```python
from build123d import *

# Parameters (mm, degrees)
F1_DEPTH      = 13
F3_W          = 5.624003956
F3_H          = 13
F4_DEPTH      = 0.5
F6_DEPTH      = 9
F8_W          = 1.375
F8_H          = 2.5
F9_DEPTH      = 0.5
F10_R         = 2
F11_R         = 1
F12_T1_DEPTH  = 14.5
F13_T1_DEPTH  = 0.5
F13_T6_DEPTH  = 0.5
F13_S7_R      = 1.95289555
F13_T8_DEPTH  = 2
F13_T12_DEPTH = 0.5
F13_S13_R     = 1.95289555
F13_T14_DEPTH = 2


# Not quite as in the source:
# - a fillet or chamfer that OpenCascade refuses, or shapes differently, is made with other operations: its cross-section is extruded or revolved along the edge and cut away or added


with BuildPart() as f1:
    # F0 (on Front) → F1 (new body)
    with BuildSketch(Plane.XZ):
        with BuildLine():
            Line((-0.1891016816, 7.3390506263), (-0.5721239031, 7.6604444312))
            Line((-0.5721239031, 7.6604444312), (-4.3080067621, 3.2081926126))
            ThreePointArc((-4.3080067621, 3.2081926126), (-4.5819264222, 1.1275662273), (-2.812001978, 0))
            Line((-2.812001978, 0), (0, 0))
            Line((0, 0), (0, 0.5))
            Line((0, 0.5), (-2.812001978, 0.5))
            ThreePointArc((-2.812001978, 0.5), (-4.1287725287, 1.3388753582), (-3.9249845405, 2.8867988077))
            Line((-3.9249845405, 2.8867988077), (-0.1891016816, 7.3390506263))
        make_face()
        with BuildLine():
            Line((0, 0.5), (0, 0))
            Line((0, 0), (2.812001978, 0))
            ThreePointArc((2.812001978, 0), (4.5819264222, 1.1275662273), (4.3080067621, 3.2081926126))
            Line((4.3080067621, 3.2081926126), (0.5721239031, 7.6604444312))
            Line((0.5721239031, 7.6604444312), (0.1891016816, 7.3390506263))
            Line((0.1891016816, 7.3390506263), (3.9249845405, 2.8867988077))
            ThreePointArc((3.9249845405, 2.8867988077), (4.1287725287, 1.3388753582), (2.812001978, 0.5))
            Line((2.812001978, 0.5), (0, 0.5))
        make_face()
    extrude(amount=-F1_DEPTH)

    # F3 (on offset) → F4 (join, through all)
    with BuildSketch(Plane(origin=(0, 0, 0), x_dir=(1, 0, 0), z_dir=(0, 0, -1))):
        with Locations((0, -6.5)):
            Rectangle(F3_W, F3_H)
        with BuildLine():
            Line((-2.812001978, 0), (2.812001978, 0))
            Line((2.812001978, 0), (4.4072171914, 0.6821090398))
            ThreePointArc((4.4072171914, 0.6821090398), (4.4747132661, 0.7384715991), (4.5, 0.8226917824))
            Line((4.5, 0.8226917824), (4.5, 15))
            Line((4.5, 15), (-4.5, 15))
            Line((-4.5, 15), (-4.5, 0.8226917824))
            ThreePointArc((-4.5, 0.8226917824), (-4.4747132661, 0.7384715991), (-4.4072171914, 0.6821090398))
            Line((-4.4072171914, 0.6821090398), (-2.812001978, 0))
        make_face()
    extrude(amount=-F4_DEPTH)

    # F5 (on face) → F6 (join, through all)
    with BuildSketch(Plane.YZ.offset(4.5)):
        Polygon((-22.4330127019, -11.874355653), (-22, -12.124355653), (-15, 0), (-15, 0.5), (-15.2886751346, 0.5), align=None)
    extrude(amount=-F6_DEPTH)

    # F8 (on offset) → F9 (join, through all)
    with BuildSketch(Plane(origin=(0, -11.6830127019, 6.7451905284), x_dir=(1, 0, 0), z_dir=(0, -0.8660254038, 0.5))):
        with Locations((-5.1875, -10.2113248654)):
            Rectangle(F8_W, F8_H)
        with BuildLine():
            Line((-5.875, -11.4613248654), (-5.875, -8.9613248654))
            Line((-5.875, -8.9613248654), (-7.25, -8.9613248654))
            ThreePointArc((-7.25, -8.9613248654), (-8.5, -10.2113248654), (-7.25, -11.4613248654))
            Line((-7.25, -11.4613248654), (-5.875, -11.4613248654))
        make_face()
        Polygon((4.5, -7.2113248654), (-4.5, -7.2113248654), (-4.5, -8.9613248654), (-4.5, -11.4613248654), (-4.5, -13.2113248654), (4.5, -13.2113248654), (4.5, -11.4613248654), (5.875, -11.4613248654), (5.875, -8.9613248654), (4.5, -8.9613248654), align=None)
        with BuildLine():
            Line((7.25, -8.9613248654), (5.875, -8.9613248654))
            Line((5.875, -8.9613248654), (5.875, -11.4613248654))
            Line((5.875, -11.4613248654), (7.25, -11.4613248654))
            ThreePointArc((7.25, -11.4613248654), (8.5, -10.2113248654), (7.25, -8.9613248654))
        make_face()
    extrude(amount=-F9_DEPTH)

    # F10
    f10_edges = [f1.edges().sort_by_distance(p)[0] for p in [
        (4.5, -22.216506, -11.999356),
        (-4.5, -22.216506, -11.999356),
    ]]
    fillet(f10_edges, radius=F10_R)

    # F11
    f11_edges = [f1.edges().sort_by_distance(p)[0] for p in [
        (0, -15.288675, 0.5),
        (0, -15, 0),
    ]]
    fillet(f11_edges, radius=F11_R)

    # F12: fillet of radius 0.3 on 4 edges, made by hand

    # F12_s2 → F12_t1 (cut)
    with BuildSketch(Plane.XZ.offset(-13.75)):
        with BuildLine():
            ThreePointArc((0.4189150145, 7.5318869093), (0.312892888, 7.3282202991), (0.3819379645, 7.1092372934))
            Line((0.3819379645, 7.1092372934), (0.1891016816, 7.3390506263))
            Line((0.1891016816, 7.3390506263), (0.4189150145, 7.5318869093))
        make_face()
        with BuildLine():
            ThreePointArc((-0.3819379645, 7.1092372934), (-0.312892888, 7.3282202991), (-0.4189150145, 7.5318869093))
            Line((-0.4189150145, 7.5318869093), (-0.1891016816, 7.3390506263))
            Line((-0.1891016816, 7.3390506263), (-0.3819379645, 7.1092372934))
        make_face()
        with BuildLine():
            ThreePointArc((0.764960186, 7.4306310983), (0.5612935759, 7.5366532248), (0.3423105702, 7.4676081483))
            Line((0.3423105702, 7.4676081483), (0.5721239031, 7.6604444312))
            Line((0.5721239031, 7.6604444312), (0.764960186, 7.4306310983))
        make_face()
        with BuildLine():
            ThreePointArc((-0.3423105702, 7.4676081483), (-0.5612935759, 7.5366532248), (-0.764960186, 7.4306310983))
            Line((-0.764960186, 7.4306310983), (-0.5721239031, 7.6604444312))
            Line((-0.5721239031, 7.6604444312), (-0.3423105702, 7.4676081483))
        make_face()
    extrude(amount=F12_T1_DEPTH, mode=Mode.SUBTRACT)

    # F13: fillet of radius 0.2 on 6 edges, made by hand

    # F13_s2 → F13_t1 (join)
    with BuildSketch(Plane(origin=(0, -11.6830127019, 6.7451905284), x_dir=(1, 0, 0), z_dir=(0, 0.8660254038, -0.5))):
        with BuildLine():
            ThreePointArc((-4.5, 8.7613248654), (-4.5585786438, 8.9027462216), (-4.7, 8.9613248654))
            Line((-4.7, 8.9613248654), (-4.5, 8.9613248654))
            Line((-4.5, 8.9613248654), (-4.5, 8.7613248654))
        make_face()
        with BuildLine():
            ThreePointArc((-4.7, 11.4613248654), (-4.5585786438, 11.5199035092), (-4.5, 11.6613248654))
            Line((-4.5, 11.6613248654), (-4.5, 11.4613248654))
            Line((-4.5, 11.4613248654), (-4.7, 11.4613248654))
        make_face()
        with BuildLine():
            ThreePointArc((4.5, 8.7613248654), (4.5585786438, 8.9027462216), (4.7, 8.9613248654))
            Line((4.7, 8.9613248654), (4.5, 8.9613248654))
            Line((4.5, 8.9613248654), (4.5, 8.7613248654))
        make_face()
        with BuildLine():
            ThreePointArc((4.7, 11.4613248654), (4.5585786438, 11.5199035092), (4.5, 11.6613248654))
            Line((4.5, 11.6613248654), (4.5, 11.4613248654))
            Line((4.5, 11.4613248654), (4.7, 11.4613248654))
        make_face()
    extrude(amount=F13_T1_DEPTH)


with BuildPart() as f13_tool4:
    # F13_s5 → F13_t6 (new body)
    with BuildSketch(Plane.XY):
        with BuildLine():
            ThreePointArc((3.7097957982, -0.3838938316), (3.5924961377, -0.159867509), (3.7884282258, 0))
            Line((3.7884282258, 0), (2.812001978, 0))
            Line((2.812001978, 0), (3.7097957982, -0.3838938316))
        make_face()
    extrude(amount=F13_T6_DEPTH)

    # F13_s7 → F13_t8 (intersect, symmetric)
    with BuildSketch(Plane.XZ.offset(0.2)):
        with Locations((2.812001978, 1.95289555)):
            Circle(F13_S7_R)
    extrude(amount=F13_T8_DEPTH, both=True, mode=Mode.INTERSECT)


with BuildPart() as f1_1:
    add(f1.part)

    # F13_t3: union F13_tool4
    add(f13_tool4.part)


with BuildPart() as f13_tool10:
    # F13_s11 → F13_t12 (new body)
    with BuildSketch(Plane.XY):
        with BuildLine():
            ThreePointArc((-3.7097957982, -0.3838938316), (-3.5924961377, -0.159867509), (-3.7884282258, 0))
            Line((-3.7884282258, 0), (-2.812001978, 0))
            Line((-2.812001978, 0), (-3.7097957982, -0.3838938316))
        make_face()
    extrude(amount=F13_T12_DEPTH)

    # F13_s13 → F13_t14 (intersect, symmetric)
    with BuildSketch(Plane.XZ.offset(0.2)):
        with Locations((-2.812001978, 1.95289555)):
            Circle(F13_S13_R)
    extrude(amount=F13_T14_DEPTH, both=True, mode=Mode.INTERSECT)


with BuildPart() as f1_2:
    add(f1_1.part)

    # F13_t9: union F13_tool10
    add(f13_tool10.part)


solid = f1_2.part
```
Input: part model. Units: mm. Frame: model coordinates. A direction names the side the tool comes from. Round coordinates to 2 decimals unless told otherwise and drop trailing zeros. Order: outer loops, then holes, each group sorted by start corner. A loop starts at its lowest first (then second) coordinate and runs counter-clockwise, first axis right, second up. Notation, with made-up numbers: (15.25, -23.75) - (32.25, -23.75) arc R20 cw to (32.25, -1.75) - close; hole circle Ø5 at (36, 22.25). An arc over 180 degrees is marked (long way). One line per question, with ' | ' between items. Start each with the question number.
1) Ray query, probe 1 along Z at (x, y) = (-0.25, -10); probe 2 along Z at (x, y) = (-0.5, 11); probe 3 along X at (y, z) = (3, 3). Return the intervals inside material, ascending.
2) Pull-direction query (Z, two-part tool) for faces 1 (the flat face through (2.56, 6.41, 5.29)), 2 (the cylindrical face through (-4.12, 6.41, 1.32)), 3 (the flat face through (4.5, -8.5, 0.2)); classes: +Z half, -Z half, draft (parallel to the pull), parting line (faces both ways), or undercut.
3) Cut plane C-C, the plane x = -5.25. Return the cut outline in (y, z).
4) Cut plane A-A, the plane y = 5. Return the cut outline in (x, z).
5) Cut plane D-D, the plane z = 5.25. Return the cut outline in (x, y), then the cut area to 3 significant figures.
6) Cut plane B-B, the plane z = 2.5. Return the cut outline in (x, y).
7) Contact query for flat-ended pins moving along their axis: P1, Ø10, axis at x = -2.5, z = 4, coming from the -Y side; P2, Ø6, axis at x = -1, y = -11.5, coming from the +Z side; P3, Ø10, axis at x = 6, y = 7.5, coming from the -Z side; P4, Ø6, axis at y = -18, z = 0.5, coming from the -X side. Output: stop coordinate, or through.
8) Set-up query: faces 4 (the flat face through (0, -4, 0.5)), 5 (the flat face through (-2.51, 6.41, 5.35)), 6 (the cylindrical face through (4.14, 6.41, 1.36)). Return all of +Z, -Z, +X, -X, +Y, -Y with unobstructed straight access to the full face (end or side cutting, diameter ignored); none if empty.
Worked out:
1) probe 1: z = 0 to 0.5 | probe 2: z = 0 to 0.5, 6.97 to 7.54 | probe 3: x = -4.46 to -3.83, 3.83 to 4.46
2) face 1: +Z half | face 2: undercut | face 3: draft
3) outline: (-17.41, -3.18) - (-16.98, -3.43) - (-15.73, -1.27) - (-16.16, -1.02) - close
4) outline: (-4.31, 3.21) arc R1.95 ccw to (-2.81, 0) - (2.81, 0) arc R1.95 ccw to (4.31, 3.21) - (0.76, 7.43) arc R0.3 ccw to (0.38, 7.5) arc R0.3 ccw to (0.38, 7.11) - (3.92, 2.89) arc R1.45 cw to (2.81, 0.5) - (-2.81, 0.5) arc R1.45 cw to (-3.92, 2.89) - (-0.38, 7.11) arc R0.3 ccw to (-0.38, 7.5) arc R0.3 ccw to (-0.76, 7.43) - close
5) outline: (-2.59, 0) - (-1.94, 0) - (-1.94, 13) - (-2.59, 13) - close; (1.94, 0) - (2.59, 0) - (2.59, 13) - (1.94, 13) - close | area: 17.0 mm^2
6) outline: (-4.69, 0) - (-4.16, 0) - (-4.16, 13) - (-4.69, 13) - close; (4.16, 0) - (4.69, 0) - (4.69, 13) - (4.16, 13) - close
7) P1: stops at y = -16.15 | P2: stops at z = 0.5 | P3: stops at z = 0 | P4: stops at x = -8.5
8) face 4: -Y | face 5: +Z, -X, +Y, -Y | face 6: +Y, -Y
